```python
from build123d import *

# Parameters (mm, degrees)
TAGLIO_ESTRUSIONE1_REACH = 262
SCHIZZO3_W               = 145
SCHIZZO3_H               = 100
TAGLIO_ESTRUSIONE2_DEPTH = 100
SCHIZZO4_R               = 4
TAGLIO_ESTRUSIONE3_DEPTH = 250
SCHIZZO6_W               = 70
SCHIZZO6_H               = 100
TAGLIO_ESTRUSIONE4_DEPTH = 18.0000001


with BuildPart() as part:
    # Schizzo1 → Rivoluzione1 (revolve)
    with BuildSketch(Plane.XY, mode=Mode.PRIVATE) as rivoluzione1_sk:
        Polygon((-21.082480081, 47.728392405), (93.917519919, 47.728392405), (93.917519919, -152.271607595), (43.917519919, -212.271607595), (-21.082480081, -212.271607595), align=None)
    revolve(rivoluzione1_sk.sketch.rotate(Axis((-21.082480081, 47.728392405, 0), (0, -1, 0)), 180), axis=Axis((-21.082480081, 47.728392405, 0), (0, -1, 0)))  # turned: the seam where the file's is

    # Taglio-Estrusione1: up to this cone (the profile starts inside it)
    taglio_estrusione1_end = Plane(origin=(-21.082480081, 47.728392, 0), z_dir=(0, 1, 0)).offset(-337.999998595) * Cone(1e-06, 735.13888827, 882.166664924, align=(Align.CENTER, Align.CENTER, Align.MIN), mode=Mode.PRIVATE)
    # Schizzo2 → Taglio-Estrusione1 (cut, up to the surface)
    with BuildSketch(Plane(origin=(0, 47.728392405, 0), x_dir=(1, 0, 0), z_dir=(0, 1, 0)), mode=Mode.PRIVATE) as taglio_estrusione1_sk1:
        with BuildLine():
            Line((60.639027234, 58.610597259), (72.534951309, 66.78904506))
            ThreePointArc((72.534951309, 66.78904506), (73.682341202, 65.150814632), (74.8010666, 63.492877363))
            Line((74.8010666, 63.492877363), (62.905142526, 55.314429562))
            ThreePointArc((62.905142526, 55.314429562), (55.621352222, 52.733884708), (60.639027234, 58.610597259))
        make_face()
    taglio_estrusione1_tool1 = extrude(taglio_estrusione1_sk1.sketch, amount=-TAGLIO_ESTRUSIONE1_REACH, mode=Mode.PRIVATE) & taglio_estrusione1_end
    add(taglio_estrusione1_tool1.solids().sort_by_distance((63.650663, 47.728392, -58.254036))[0], mode=Mode.SUBTRACT)
    # Schizzo2 → Taglio-Estrusione1 (cut, up to the surface)
    with BuildSketch(Plane(origin=(0, 47.728392405, 0), x_dir=(1, 0, 0), z_dir=(0, 1, 0)), mode=Mode.PRIVATE) as taglio_estrusione1_sk2:
        with BuildLine():
            Line((37.528117178, -81.721507315), (45.706564979, -93.617431389))
            ThreePointArc((45.706564979, -93.617431389), (44.068334551, -94.764821283), (42.410397283, -95.883546681))
            Line((42.410397283, -95.883546681), (34.231949481, -83.987622606))
            ThreePointArc((34.231949481, -83.987622606), (31.651404628, -76.703832303), (37.528117178, -81.721507315))
        make_face()
    taglio_estrusione1_tool2 = extrude(taglio_estrusione1_sk2.sketch, amount=-TAGLIO_ESTRUSIONE1_REACH, mode=Mode.PRIVATE) & taglio_estrusione1_end
    add(taglio_estrusione1_tool2.solids().sort_by_distance((37.171556, 47.728392, 84.733143))[0], mode=Mode.SUBTRACT)
    # Schizzo2 → Taglio-Estrusione1 (cut, up to the surface)
    with BuildSketch(Plane(origin=(0, 47.728392405, 0), x_dir=(1, 0, 0), z_dir=(0, 1, 0)), mode=Mode.PRIVATE) as taglio_estrusione1_sk3:
        with BuildLine():
            Line((-102.803987396, -58.610597259), (-114.69991147, -66.78904506))
            ThreePointArc((-114.69991147, -66.78904506), (-115.847301364, -65.150814632), (-116.966026762, -63.492877363))
            Line((-116.966026762, -63.492877363), (-105.070102687, -55.314429562))
            ThreePointArc((-105.070102687, -55.314429562), (-97.786312384, -52.733884708), (-102.803987396, -58.610597259))
        make_face()
    taglio_estrusione1_tool3 = extrude(taglio_estrusione1_sk3.sketch, amount=-TAGLIO_ESTRUSIONE1_REACH, mode=Mode.PRIVATE) & taglio_estrusione1_end
    add(taglio_estrusione1_tool3.solids().sort_by_distance((-105.815623, 47.728392, 58.254036))[0], mode=Mode.SUBTRACT)
    # Schizzo2 → Taglio-Estrusione1 (cut, up to the surface)
    with BuildSketch(Plane(origin=(0, 47.728392405, 0), x_dir=(1, 0, 0), z_dir=(0, 1, 0)), mode=Mode.PRIVATE) as taglio_estrusione1_sk4:
        with BuildLine():
            Line((-79.69307734, 81.721507315), (-87.871525141, 93.617431389))
            ThreePointArc((-87.871525141, 93.617431389), (-86.233294713, 94.764821283), (-84.575357444, 95.883546681))
            Line((-84.575357444, 95.883546681), (-76.396909643, 83.987622606))
            ThreePointArc((-76.396909643, 83.987622606), (-73.816364789, 76.703832303), (-79.69307734, 81.721507315))
        make_face()
    taglio_estrusione1_tool4 = extrude(taglio_estrusione1_sk4.sketch, amount=-TAGLIO_ESTRUSIONE1_REACH, mode=Mode.PRIVATE) & taglio_estrusione1_end
    add(taglio_estrusione1_tool4.solids().sort_by_distance((-79.336516, 47.728392, -84.733143))[0], mode=Mode.SUBTRACT)

    # Schizzo3 → Taglio-Estrusione2 (cut)
    with BuildSketch(Plane(origin=(0, 47.728392405, 0), x_dir=(1, 0, 0), z_dir=(0, 1, 0))):
        with Locations((-21.082480081, 0)):
            Rectangle(SCHIZZO3_W, SCHIZZO3_H)
    extrude(amount=-TAGLIO_ESTRUSIONE2_DEPTH, mode=Mode.SUBTRACT)

    # Schizzo4 → Taglio-Estrusione3 (cut)
    with BuildSketch(Plane(origin=(0, 47.728392405, 0), x_dir=(1, 0, 0), z_dir=(0, 1, 0))):
        with Locations(Location((-71.082480081, 0, 0), (0, 0, 180))):  # turned: the seam where the file's is
            Circle(SCHIZZO4_R)
        with Locations(Location((28.917519919, 0, 0), (0, 0, 180))):  # turned: the seam where the file's is
            Circle(SCHIZZO4_R)
    extrude(amount=-TAGLIO_ESTRUSIONE3_DEPTH, mode=Mode.SUBTRACT)

    # Schizzo6 → Taglio-Estrusione4 (cut, through all)
    with BuildSketch(Plane.XY.offset(98)):
        with Locations((-21.082480081, -52.271607595)):
            Rectangle(SCHIZZO6_W, SCHIZZO6_H)
    extrude(amount=TAGLIO_ESTRUSIONE4_DEPTH, mode=Mode.SUBTRACT)


solid = part.part
```
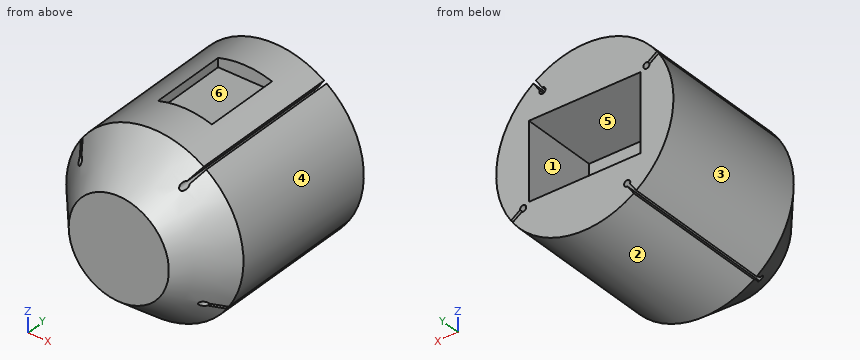
The listing builds one solid part. Answer for the finished solid, in the listing's coordinates (mm). Face numbers are marked on the shaded views. A direction names the side the tool comes from. Give positions to 0.01 mm unless a question says otherwise; leave off trailing zeros. Write each loop counter-clockwise with the first axis right and the second up, starting at its lowest first coordinate (ties: lowest second). Pieces come first, ordered by that corner, then holes. Notation, with made-up numbers: (62.25, -2) -> (73.25, -2) arc R29 cw to (73.25, 30) -> close; hole circle Ø11 at (0, -36.75). An arc over 180 degrees is marked (long way). Write item = value, one per line. Start each with the question number.
1) Determine the mould class of the marked faces 1, 2 and 3 for opening direction Z: +Z half, -Z half, draft (parallel to the pull), parting line (faces both ways), or undercut.
2) The part is cut by section C-C, the plane z = 0. Determine the outline of the cut face in (x, y), and give its area (3 significant figures).
3) The part is cut by section B-B, the plane y = -124.5. Determine the outline of the cut face in (x, z), and give its area (3 significant figures).
4) Which of the six approach directions +Z, -Z, +X, -X, +Y, -Y give full straight-line access (tool end or side, diameter ignored) to the marked faces 4, 5 and 6?
5) Each of these flat-tipped pins is pushed along its axis until it touches: pin 1 (2.5 mm diameter, centred on x = 30.5, z = 2, fed in from +Y); pin 2 (9 mm diameter, centred on x = -76.08, z = -80, fed in from -Y); pin 3 (9 mm diameter, centred on y = -35, z = 106.5, fed in from -X). Where does it stop, or does it pass through?
6) Straight lines are drawn through the part: line 1 along Z through (x, y) = (-21.5, -26.5); line 2 along Y through (x, z) = (-40, 35); line 3 along X through (y, z) = (-7, -23). For each, find the intervals that lie inside material, in ascending order.
7) The part is cut by section A-A, the plane y = 8. Determine the outline of the cut face in (x, z).
Solutions:
q1.face_1 = undercut
q1.face_2 = -Z half
q1.face_3 = parting line
q2.outline = (-136.08, -152.27) -> (-86.08, -212.27) -> (43.92, -212.27) -> (93.92, -152.27) -> (93.92, 47.73) -> (51.42, 47.73) -> (51.42, -52.27) -> (32.92, -52.27) -> (32.92, -202.27) -> (24.92, -202.27) -> (24.92, -52.27) -> (-67.08, -52.27) -> (-67.08, -202.27) -> (-75.08, -202.27) -> (-75.08, -52.27) -> (-93.58, -52.27) -> (-93.58, 47.73) -> (-136.08, 47.73) -> close
q2.area = 39,900 mm²
q3.outline = (-116.97, 63.49) arc R115 ccw to (-87.87, -93.62) -> (-79.69, -81.72) arc R4 cw (long way) to (-76.4, -83.99) -> (-84.58, -95.88) arc R115 ccw to (72.53, -66.79) -> (60.64, -58.61) arc R4 cw (long way) to (62.91, -55.31) -> (74.8, -63.49) arc R115 ccw to (45.71, 93.62) -> (37.53, 81.72) arc R4 cw (long way) to (34.23, 83.99) -> (42.41, 95.88) arc R115 ccw to (-114.7, 66.79) -> (-102.8, 58.61) arc R4 cw (long way) to (-105.07, 55.31) -> close; hole circle Ø8 at (-71.08, 0); hole circle Ø8 at (28.92, 0)
q3.area = 41,000 mm²
q4.face_4 = +X, +Y, -Y
q4.face_5 = +Y
q4.face_6 = +Z
q5.pin_1 = -202.27
q5.pin_2 = -179.17
q5.pin_3 = -74.2
q6.line_1 = -115 to -50, 50 to 98
q6.line_2 = -212.27 to -52.27
q6.line_3 = -133.76 to -93.58, 51.42 to 91.59
q7.outline = (-116.97, 63.49) arc R115 ccw to (-87.87, -93.62) -> (-79.69, -81.72) arc R4 cw (long way) to (-76.4, -83.99) -> (-84.58, -95.88) arc R115 ccw to (72.53, -66.79) -> (60.64, -58.61) arc R4 cw (long way) to (62.91, -55.31) -> (74.8, -63.49) arc R115 ccw to (45.71, 93.62) -> (37.53, 81.72) arc R4 cw (long way) to (34.23, 83.99) -> (42.41, 95.88) arc R115 ccw to (-114.7, 66.79) -> (-102.8, 58.61) arc R4 cw (long way) to (-105.07, 55.31) -> close; hole (-93.58, -50) -> (51.42, -50) -> (51.42, 50) -> (-93.58, 50) -> close
